The listing builds one solid part. Answer for the finished solid, in the listing's coordinates (mm). A direction names the side the tool comes from. Coordinates: 2 decimals unless noted, no trailing zeros. Order: outer loops, then holes, each group sorted by start corner. A loop starts at its lowest first (then second) coordinate and runs counter-clockwise, first axis right, second up. Notation, with made-up numbers: (-15, -6) - (42, -6) arc R9 ccw to (42, 10) - close; hole circle Ø4 at (26, 41). An arc over 180 degrees is marked (long way). Use a Markdown table: item, result. Add a question column.
Item 1: The mould has two halves that part along Y. Classify faces 1 (the flat face through (-0.2, 6.5, 2.5)), 2 (the flat face through (0, 12.5, 1)), 3 (the flat face through (0, 11, 3)): released by +Y, released by -Y, zero draft, split by the parting line, or undercut.
Item 2: Find the intervals of material crossed by line 1 along Y through (x, z) = (2.25, 2.05); line 2 along Z through (x, y) = (-6.75, -2.25), in increasing order.
Item 3: The part is cut by section B-B, the plane x = 1.25. Give the vertices of the cut face in (y, z).
Item 4: The part is cut by section C-C, the plane y = -1. Give the vertices of the cut face in (x, z), then the cut area to 3 significant figures.
Item 5: The part is cut by section A-A, the plane z = 2.3. Give the vertices of the cut face in (x, y).
Item 6: A flat-ended cylindrical pin translates along its axis: P1, Ø1.5, axis at x = -5.5, y = -6.5, coming from the +Z side. Find the tip coordinate at first contact, or state that the pin passes through.
Item 7: For faces 4 (the flat face through (-0.2, 8.5, 2.5)), 5 (the flat face through (0, 0, 3)), determine the directions among +Z, -Z, +X, -X, +Y, -Y from which every point of the face is accessible in a straight line to the end or side of a thin tool.
from build123d import *

# Parameters (mm, degrees)
F0_W     = 25
F0_H     = 25
F1_DEPTH = 3
F2_W     = 25
F2_H     = 2
F3_DEPTH = 1
F2_H_2   = 3
F2_H_3   = 4
F2_H_4   = 5


with BuildPart() as f1:
    # F0 (on Top) → F1 (new body)
    with BuildSketch(Plane.XY):
        Rectangle(F0_W, F0_H)
    extrude(amount=F1_DEPTH)


with BuildPart() as f3:
    # F2 (on face) → F3 (new body)
    with BuildSketch(Plane.XY.offset(3)):
        with Locations((0, 7.5)):
            Rectangle(F2_W, F2_H)
    extrude(amount=-F3_DEPTH)


with BuildPart() as f3b:
    # F2 (on face) → F3, piece 2 (new body)
    with BuildSketch(Plane.XY.offset(3)):
        with Locations((0, 2.5)):
            Rectangle(F2_W, F2_H_2)
    extrude(amount=-F3_DEPTH)


with BuildPart() as f3c:
    # F2 (on face) → F3, piece 3 (new body)
    with BuildSketch(Plane.XY.offset(3)):
        with Locations((0, -2.5)):
            Rectangle(F2_W, F2_H_3)
    extrude(amount=-F3_DEPTH)


with BuildPart() as f3d:
    # F2 (on face) → F3, piece 4 (new body)
    with BuildSketch(Plane.XY.offset(3)):
        with Locations((0, -7.5)):
            Rectangle(F2_W, F2_H_4)
    extrude(amount=-F3_DEPTH)


with BuildPart() as f1_1:
    add(f1.part)

    # F4: cut F3, F3b, F3c, F3d
    add(f3.part, mode=Mode.SUBTRACT)
    add(f3b.part, mode=Mode.SUBTRACT)
    add(f3c.part, mode=Mode.SUBTRACT)
    add(f3d.part, mode=Mode.SUBTRACT)


solid = f1_1.part
Solution:
| question | item | result |
|---|---|---|
| 1 | face 1 | undercut |
| 1 | face 2 | released by +Y |
| 1 | face 3 | zero draft |
| 2 | line 1 | y = -12.5 to -10, -5 to -4.5, -0.5 to 1, 4 to 6.5, 8.5 to 12.5 |
| 2 | line 2 | z = 0 to 2 |
| 3 | outline | (-12.5, 0) - (12.5, 0) - (12.5, 3) - (8.5, 3) - (8.5, 2) - (6.5, 2) - (6.5, 3) - (4, 3) - (4, 2) - (1, 2) - (1, 3) - (-0.5, 3) - (-0.5, 2) - (-4.5, 2) - (-4.5, 3) - (-5, 3) - (-5, 2) - (-10, 2) - (-10, 3) - (-12.5, 3) - close |
| 4 | outline | (-12.5, 0) - (12.5, 0) - (12.5, 2) - (-12.5, 2) - close |
| 4 | area | 50.0 mm2 |
| 5 | outline | (-12.5, -12.5) - (12.5, -12.5) - (12.5, -10) - (-12.5, -10) - close; (-12.5, -5) - (12.5, -5) - (12.5, -4.5) - (-12.5, -4.5) - close; (-12.5, -0.5) - (12.5, -0.5) - (12.5, 1) - (-12.5, 1) - close; (-12.5, 4) - (12.5, 4) - (12.5, 6.5) - (-12.5, 6.5) - close; (-12.5, 8.5) - (12.5, 8.5) - (12.5, 12.5) - (-12.5, 12.5) - close |
| 6 | P1 | stops at z = 2 |
| 7 | face 4 | +Z, +X, -X |
| 7 | face 5 | +Z, +X, -X, +Y, -Y |
